Verification items for the finished model (mm, model axes). A direction names the side the tool comes from. Coordinates: 2 decimals unless noted, no trailing zeros. Loops run counter-clockwise (first coordinate to the right, second up) from the corner with the lowest first, then second, coordinate; pieces in that order, holes last.
Q1. Sectioned sample at A-A (x = 0). Enter the section's corners in (y, z), then the cut area to 3 significant figures.
Q2. Material ranges on probe 1 along Y at (x, z) = (0, 11.6); probe 2 along Y at (x, z) = (0, 10); probe 3 along Y at (x, z) = (5, 11.2) (3 decimals), recorded low to high.
Q3. Sectioned sample at B-B (y = 0). Enter the section's corners in (x, z).
Q4. Sectioned sample at C-C (x = -10). Enter the section's corners in (y, z), then the cut area to 3 significant figures.
Q5. Sectioned sample at D-D (y = -4.5). Enter the section's corners in (x, z), then the cut area to 3 significant figures.
Q6. Go/stop test with flat-tipped pins: P1, Ø1, axis at x = 5, y = -8.66, coming from the -Z side; P2, Ø2, axis at x = 3.5, z = 11, coming from the +Y side; P3, Ø9.5, axis at x = 0, y = 0, coming from the +Z side; P4, Ø1, axis at y = -2, z = 10.5, coming from the -X side. Record where each tip stops, or that it passes through.
Q7. Access from +Z, -Z, +X, -X, +Y, -Y to the whole of each face (thin tool, end or side, straight path). Record for faces 1 (the face through (5, 9, 9.75)), 2 (the face through (7, 0, 9.5)), 3 (the face through (-1.19, -5.37, 9.76)).
Q8. Mould release check, pull along X, two halves, no side actions. Record for faces 4 (the face through (-3, -5, 9)), 5 (the face through (-10.6, 0, 11.3)), 6 (the face through (-3.47, -15.62, 11.1)), 7 (the face through (4.922, 9.255, 11.271)): +X half, -X half, draft (parallel to the pull), parting line (faces both ways), or undercut.
```python
from build123d import *

# Parameters (mm, degrees)
SKETCH_1_R          = 16
EXTRUDE_1_DEPTH     = 9
SKETCH_2_R          = 6
EXTRUDE_2_DEPTH     = 0.5
SKETCH_3_R          = 16
EXTRUDE_3_DEPTH     = 3.25
SKETCH_4_R          = 5.5
EXTRUDE_4_DEPTH     = 2.25
SKETCH_5_R          = 3
CUT_EXTRUDE_1_DEPTH = 26.25
SKETCH_6_R          = 8
SKETCH_6_R_2        = 5.5
CUT_EXTRUDE_2_DEPTH = 2.25
SKETCH_7_R          = 0.6
CUT_EXTRUDE_3_DEPTH = 6
SKETCH_8_R          = 0.6
CUT_EXTRUDE_4_DEPTH = 3
SKETCH_9_R          = 28.808997231
CUT_EXTRUDE_5_DEPTH = 9
SKETCH_10_R         = 5.5
CUT_EXTRUDE_6_DEPTH = 9


with BuildPart() as part:
    # 草图1 → 凸台-拉伸1 (new body)
    with BuildSketch(Plane.XY):
        Circle(SKETCH_1_R)
    extrude(amount=EXTRUDE_1_DEPTH)

    # 草图2 → 凸台-拉伸2 (add)
    with BuildSketch(Plane.XY.offset(9)):
        Circle(SKETCH_2_R)
    extrude(amount=EXTRUDE_2_DEPTH)

    # 草图3 → 凸台-拉伸3 (add)
    with BuildSketch(Plane.XY.offset(9.5)):
        Circle(SKETCH_3_R)
    extrude(amount=EXTRUDE_3_DEPTH)

    # 草图4 → 凸台-拉伸4 (add)
    with BuildSketch(Plane.XY.offset(12.75)):
        Circle(SKETCH_4_R)
    extrude(amount=EXTRUDE_4_DEPTH)

    # 草图5 → 切除-拉伸1 (cut)
    with BuildSketch(Plane.XY.offset(15)):
        Circle(SKETCH_5_R)
    extrude(amount=-CUT_EXTRUDE_1_DEPTH, mode=Mode.SUBTRACT)

    # 草图6 → 切除-拉伸2 (cut)
    with BuildSketch(Plane.XY.offset(12.75)):
        Circle(SKETCH_6_R)
        Circle(SKETCH_6_R_2, mode=Mode.SUBTRACT)
    extrude(amount=-CUT_EXTRUDE_2_DEPTH, mode=Mode.SUBTRACT)

    # 草图7 → 切除-拉伸3 (cut)
    with BuildSketch(Plane(origin=(0, 0, 0), x_dir=(-1, 0, 0), z_dir=(0, 0, -1))):
        with Locations((8.660254038, 5)):
            Circle(SKETCH_7_R)
        with Locations((-8.660254038, 5)):
            Circle(SKETCH_7_R)
        with Locations((0, -10)):
            Circle(SKETCH_7_R)
    extrude(amount=-CUT_EXTRUDE_3_DEPTH, mode=Mode.SUBTRACT)

    # 草图8 → 切除-拉伸4 (cut)
    with BuildSketch(Plane.XY.offset(12.75)):
        with Locations((5, -8.660254038)):
            Circle(SKETCH_8_R)
        with Locations((5, 8.660254038)):
            Circle(SKETCH_8_R)
        with Locations((-10, 0)):
            Circle(SKETCH_8_R)
    extrude(amount=-CUT_EXTRUDE_4_DEPTH, mode=Mode.SUBTRACT)

    # 草图9 → 切除-拉伸5 (cut)
    with BuildSketch(Plane(origin=(0, 0, 0), x_dir=(-1, 0, 0), z_dir=(0, 0, -1))):
        Circle(SKETCH_9_R)
    extrude(amount=-CUT_EXTRUDE_5_DEPTH, mode=Mode.SUBTRACT)

    # 草图10 → 切除-拉伸6 (cut)
    with BuildSketch(Plane.XY.offset(15)):
        Circle(SKETCH_10_R)
    extrude(amount=-CUT_EXTRUDE_6_DEPTH, mode=Mode.SUBTRACT)


solid = part.part
```
Geometry check:
1. outline: (-16, 9.5) - (-6, 9.5) - (-6, 9) - (-5.5, 9) - (-5.5, 10.5) - (-8, 10.5) - (-8, 12.75) - (-16, 12.75) - close; (5.5, 9) - (6, 9) - (6, 9.5) - (16, 9.5) - (16, 12.75) - (8, 12.75) - (8, 10.5) - (5.5, 10.5) - close
1. area: 57.5 mm2
2. probe 1: y = -16 to -8, 8 to 16
2. probe 2: y = -16 to -5.5, 5.5 to 16
2. probe 3: y = -15.199 to -9.26, -8.06 to -6.245, 6.245 to 8.06, 9.26 to 15.199
3. outline: (-16, 9.5) - (-6, 9.5) - (-6, 9) - (-5.5, 9) - (-5.5, 10.5) - (-8, 10.5) - (-8, 12.75) - (-9.4, 12.75) - (-9.4, 9.75) - (-10.6, 9.75) - (-10.6, 12.75) - (-16, 12.75) - close; (5.5, 9) - (6, 9) - (6, 9.5) - (16, 9.5) - (16, 12.75) - (8, 12.75) - (8, 10.5) - (5.5, 10.5) - close
4. outline: (-12.49, 9.5) - (12.49, 9.5) - (12.49, 12.75) - (0.6, 12.75) - (0.6, 9.75) - (-0.6, 9.75) - (-0.6, 12.75) - (-12.49, 12.75) - close
4. area: 77.6 mm2
5. outline: (-15.35, 9.5) - (-3.97, 9.5) - (-3.97, 9) - (-3.16, 9) - (-3.16, 10.5) - (-6.61, 10.5) - (-6.61, 12.75) - (-15.35, 12.75) - close; (3.16, 9) - (3.97, 9) - (3.97, 9.5) - (15.35, 9.5) - (15.35, 12.75) - (6.61, 12.75) - (6.61, 10.5) - (3.16, 10.5) - close
5. area: 64.5 mm2
6. P1: stops at z = 9.5
6. P2: stops at y = 15.8
6. P3: passes through
6. P4: stops at x = -15.93
7. face 1: +Z
7. face 2: -Z
7. face 3: +Z, -Z
8. face 4: draft
8. face 5: undercut
8. face 6: parting line
8. face 7: undercut
